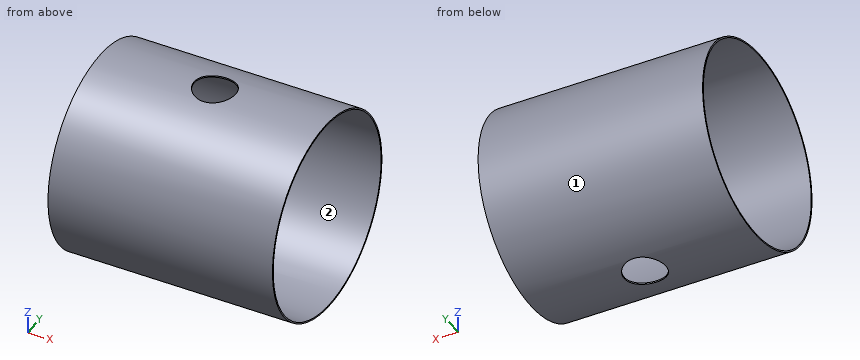
Autodesk Inventor part; units mm, degrees
ref_plane "YZ Plane" through (0, 0, 0) normal (1, 0, 0) x (0, 1, 0)
ref_plane "XZ Plane" through (0, 0, 0) normal (0, 1, 0) x (-1, 0, 0)
ref_plane "XY Plane" through (0, 0, 0) normal (0, 0, 1) x (1, 0, 0)
sketch "Sketch1" plane through (0, 0, 0) normal (1, 0, 0) x (0, 1, 0)
  circle A0 centre (0, 0) radius 72
  dimension "d0" = 144
extrude "Extrusion1" add sketch "Sketch1" along normal blind 164
sketch "Sketch2" plane through (164, 0, 0) normal (1, 0, 0) x (0, 0, -1)
  circle A0 centre (0, 0) radius 71
  dimension "d3" = 142
extrude "Extrusion2" cut sketch "Sketch2" against normal blind 300
sketch "Sketch3" plane through (0, 0, 0) normal (0, 0, 1) x (1, 0, 0)
  line L0 (0, 0) -> (82, 0)
  circle A0 centre (82, 0) radius 15
  dimension "d6" = 82
  dimension "d7" = 30
extrude "Extrusion3" cut sketch "Sketch3" along normal mid plane 164
properties part number "Shield Center"
Could you check a few things on this model? Use its own coordinates, in mm. Face numbers are marked on the shaded views. Coordinates: 2 decimals unless noted, no trailing zeros. Loops run counter-clockwise (first coordinate to the right, second up) from the corner with the lowest first, then second, coordinate; pieces in that order, holes last. Notation, with made-up numbers: (67, -8.5) -> (73, -8.5) arc R22 cw to (73, -1.5) -> close; hole circle Ø8 at (-21, -28.75). An arc over 180 degrees is marked (long way). Answer in a Markdown table with one row per item.
(1) Imagine slicing it at D-D (x = 134). List the corners of the cut face in (y, z) for me, plus the area to 3 significant figures.
Results found:
| item | result |
|---|---|
| outline | circle Ø144 at (0, 0); hole circle Ø142 at (0, 0) |
| area | 449 mm^2 |
(2) Will these pins go through, and if not, where does the flat tip stop? pin 1 Ø5 at (x, z) = (99.5, -26) entering from -Y; pin 2 Ø1 at (x, y) = (85, -47) entering from -Z; pin 3 Ø1.5 at (x, y) = (144.5, -44) entering from +Z.
Results found:
| item | result |
|---|---|
| pin 1 | stops at y = -68.06 |
| pin 2 | stops at z = -54.97 |
| pin 3 | stops at z = 57.56 |
(3) If I drill on probe 1 along X at (y, z) = (0, -71.2); probe 2 along Z at (x, y) = (123.5, 34); probe 3 along Z at (x, y) = (121, 22.5), over which ranges is the centre line in solid material (lowest first)?
Results found:
| item | result |
|---|---|
| probe 1 | x = 0 to 67, 97 to 164 |
| probe 2 | z = -63.47 to -62.33, 62.33 to 63.47 |
| probe 3 | z = -68.39 to -67.34, 67.34 to 68.39 |
(4) Imagine slicing it at C-C (x = 94.5). List the corners of the cut face in (y, z) for me, plus the area to 3 significant figures.
Results found:
| item | result |
|---|---|
| outline | (-8.29, -71.52) -> (-8.29, -70.51) arc R71 cw to (-8.29, 70.51) -> (-8.29, 71.52) arc R72 ccw to start; (8.29, -71.52) arc R72 ccw to (8.29, 71.52) -> (8.29, 70.51) arc R71 cw to (8.29, -70.51) -> close |
| area | 416 mm^2 |
(5) Thinking about a two-plate mould opening in Y: for the marked faces 1 and 2, which applies, released by +Y, released by -Y, zero draft, split by the parting line, or undercut?
Results found:
| item | result |
|---|---|
| face 1 | split by the parting line |
| face 2 | undercut |
